Could you check a few things on this model? Use its own coordinates, in mm. Round coordinates to 2 decimals unless told otherwise and drop trailing zeros. Write each loop counter-clockwise with the first axis right and the second up, starting at its lowest first coordinate (ties: lowest second). Pieces come first, ordered by that corner, then holes. Notation, with made-up numbers: (31, 48.5) - (83, 48.5) arc R15 ccw to (83, 56.5) - close; hole circle Ø9 at (-39, 80.5). An arc over 180 degrees is marked (long way). Write each question's results on one line, items separated by ' | '. Start each with the question number.
(1) Imagine slicing it at B-B on z = 2.2. State how many separate pieces and enclosed holes the cut face has, then the cut area to 3 significant figures.
(2) Please list where these lines run through material, in increasing order: line 1 (X direction, y = -50.5, z = 1.2); line 2 (X direction, y = 9, z = 2.4); line 3 (Y direction, x = 144, z = 0.4). Write a range as [from, to].
(3) Imagine slicing it at A-A on y = 17. Write out the boundary of the cut face in (x, z), then the cut area to 3 significant figures.
(4) Thinking about a two-plate mould opening in X: for faces 1 (the cylindrical face through (42.734, -25.896, 1.972)), 2 (the flat face through (73, -15, 4)), which applies, +X half, -X half, draft (parallel to the pull), parting line (faces both ways), or undercut?
```python
from build123d import *

# Parameters (mm, degrees)
SKETCH1_W           = 270
SKETCH1_H           = 200
SKETCH1_R           = 1.5
SKETCH1_R_2         = 10
SKETCH1_R_3         = 2.5
BOSS_EXTRUDE1_DEPTH = 4


with BuildPart() as part:
    # Sketch1 → Boss-Extrude1 (new body)
    with BuildSketch(Plane.XY):
        with Locations((74.901502586, -16.133333333)):
            Rectangle(SKETCH1_W, SKETCH1_H)
        with Locations((-32.098497414, -92.133333333)):
            Circle(SKETCH1_R, mode=Mode.SUBTRACT)
        with Locations((-17.098497414, -92.133333333)):
            Circle(SKETCH1_R, mode=Mode.SUBTRACT)
        with Locations((-32.098497414, -107.133333333)):
            Circle(SKETCH1_R, mode=Mode.SUBTRACT)
        with Locations((-47.098497414, -92.133333333)):
            Circle(SKETCH1_R, mode=Mode.SUBTRACT)
        with Locations((-32.098497414, -77.133333333)):
            Circle(SKETCH1_R, mode=Mode.SUBTRACT)
        with Locations((74.901502586, -16.133333333)):
            Circle(SKETCH1_R, mode=Mode.SUBTRACT)
        with Locations((196.901502586, -92.133333333)):
            Circle(SKETCH1_R, mode=Mode.SUBTRACT)
        with Locations((181.901502586, -77.133333333)):
            Circle(SKETCH1_R, mode=Mode.SUBTRACT)
        with Locations((181.901502586, -92.133333333)):
            Circle(SKETCH1_R, mode=Mode.SUBTRACT)
        with Locations((181.901502586, -107.133333333)):
            Circle(SKETCH1_R, mode=Mode.SUBTRACT)
        with Locations((166.901502586, -92.133333333)):
            Circle(SKETCH1_R, mode=Mode.SUBTRACT)
        with Locations((196.901502586, 59.866666667)):
            Circle(SKETCH1_R, mode=Mode.SUBTRACT)
        with Locations((181.901502586, 74.866666667)):
            Circle(SKETCH1_R, mode=Mode.SUBTRACT)
        with Locations((181.901502586, 59.866666667)):
            Circle(SKETCH1_R, mode=Mode.SUBTRACT)
        with Locations((181.901502586, 44.866666667)):
            Circle(SKETCH1_R, mode=Mode.SUBTRACT)
        with Locations((166.901502586, 59.866666667)):
            Circle(SKETCH1_R, mode=Mode.SUBTRACT)
        with Locations((-17.098497414, 59.866666667)):
            Circle(SKETCH1_R, mode=Mode.SUBTRACT)
        with Locations((-32.098497414, 74.866666667)):
            Circle(SKETCH1_R, mode=Mode.SUBTRACT)
        with Locations((-32.098497414, 59.866666667)):
            Circle(SKETCH1_R, mode=Mode.SUBTRACT)
        with Locations((-32.098497414, 44.866666667)):
            Circle(SKETCH1_R, mode=Mode.SUBTRACT)
        with Locations((-47.098497414, 59.866666667)):
            Circle(SKETCH1_R, mode=Mode.SUBTRACT)
        with Locations((181.901502586, -16.133333333)):
            Circle(SKETCH1_R, mode=Mode.SUBTRACT)
        with Locations((74.901502586, 59.866666667)):
            Circle(SKETCH1_R, mode=Mode.SUBTRACT)
        with Locations((104.901502586, -16.133333333)):
            Circle(SKETCH1_R_2, mode=Mode.SUBTRACT)
        with Locations((44.901502586, -16.133333333)):
            Circle(SKETCH1_R_2, mode=Mode.SUBTRACT)
        with Locations((-32.098497414, -16.133333333)):
            Circle(SKETCH1_R, mode=Mode.SUBTRACT)
        with Locations((74.901502586, -92.133333333)):
            Circle(SKETCH1_R, mode=Mode.SUBTRACT)
        with Locations((4.901502586, 38.866666667)):
            Circle(SKETCH1_R_3, mode=Mode.SUBTRACT)
        with Locations((54.901502586, 38.866666667)):
            Circle(SKETCH1_R_3, mode=Mode.SUBTRACT)
        with Locations((94.901502586, 38.866666667)):
            Circle(SKETCH1_R_3, mode=Mode.SUBTRACT)
        with Locations((144.901502586, 38.866666667)):
            Circle(SKETCH1_R_3, mode=Mode.SUBTRACT)
        with Locations((94.901502586, -71.133333333)):
            Circle(SKETCH1_R_3, mode=Mode.SUBTRACT)
        with Locations((144.901502586, -71.133333333)):
            Circle(SKETCH1_R_3, mode=Mode.SUBTRACT)
        with Locations((4.901502586, -71.133333333)):
            Circle(SKETCH1_R_3, mode=Mode.SUBTRACT)
        with Locations((54.901502586, -71.133333333)):
            Circle(SKETCH1_R_3, mode=Mode.SUBTRACT)
        with Locations((-45.098497414, 8.866666667)):
            Circle(SKETCH1_R, mode=Mode.SUBTRACT)
        with Locations((12.901502586, 8.866666667)):
            Circle(SKETCH1_R, mode=Mode.SUBTRACT)
        with Locations((12.901502586, -40.133333333)):
            Circle(SKETCH1_R, mode=Mode.SUBTRACT)
        with Locations((-45.098497414, -40.133333333)):
            Circle(SKETCH1_R, mode=Mode.SUBTRACT)
        with Locations((29.901502586, 35.366666667)):
            Circle(SKETCH1_R, mode=Mode.SUBTRACT)
        with Locations((87.901502586, 35.366666667)):
            Circle(SKETCH1_R, mode=Mode.SUBTRACT)
        with Locations((87.901502586, -67.633333333)):
            Circle(SKETCH1_R, mode=Mode.SUBTRACT)
        with Locations((29.901502586, -67.633333333)):
            Circle(SKETCH1_R, mode=Mode.SUBTRACT)
        with Locations((107.901502586, 33.866666667)):
            Circle(SKETCH1_R, mode=Mode.SUBTRACT)
        with Locations((187.901502586, 33.866666667)):
            Circle(SKETCH1_R, mode=Mode.SUBTRACT)
        with Locations((187.901502586, -66.133333333)):
            Circle(SKETCH1_R, mode=Mode.SUBTRACT)
        with Locations((107.901502586, -66.133333333)):
            Circle(SKETCH1_R, mode=Mode.SUBTRACT)
        with BuildLine():
            Line((183.401502586, -45.133333333), (183.401502586, -73.133333333))
            ThreePointArc((183.401502586, -73.133333333), (181.901502586, -74.633333333), (180.401502586, -73.133333333))
            Line((180.401502586, -73.133333333), (180.401502586, -45.133333333))
            ThreePointArc((180.401502586, -45.133333333), (181.901502586, -43.633333333), (183.401502586, -45.133333333))
        make_face(mode=Mode.SUBTRACT)
        with BuildLine():
            Line((-33.598497414, -45.133333333), (-33.598497414, -73.133333333))
            ThreePointArc((-33.598497414, -73.133333333), (-32.098497414, -74.633333333), (-30.598497414, -73.133333333))
            Line((-30.598497414, -73.133333333), (-30.598497414, -45.133333333))
            ThreePointArc((-30.598497414, -45.133333333), (-32.098497414, -43.633333333), (-33.598497414, -45.133333333))
        make_face(mode=Mode.SUBTRACT)
        with BuildLine():
            Line((-33.598497414, 40.866666667), (-33.598497414, 12.866666667))
            ThreePointArc((-33.598497414, 12.866666667), (-32.098497414, 11.366666667), (-30.598497414, 12.866666667))
            Line((-30.598497414, 12.866666667), (-30.598497414, 40.866666667))
            ThreePointArc((-30.598497414, 40.866666667), (-32.098497414, 42.366666667), (-33.598497414, 40.866666667))
        make_face(mode=Mode.SUBTRACT)
        with BuildLine():
            Line((180.401502586, 40.866666667), (180.401502586, 12.866666667))
            ThreePointArc((180.401502586, 12.866666667), (181.901502586, 11.366666667), (183.401502586, 12.866666667))
            Line((183.401502586, 12.866666667), (183.401502586, 40.866666667))
            ThreePointArc((183.401502586, 40.866666667), (181.901502586, 42.366666667), (180.401502586, 40.866666667))
        make_face(mode=Mode.SUBTRACT)
    extrude(amount=BOSS_EXTRUDE1_DEPTH)


solid = part.part
```
Response:
1) separate pieces: 1 | enclosed holes: 51 | area: 52,600 mm²
2) line 1: [-60.1, -33.6], [-30.6, 180.4], [183.4, 209.9] | line 2: [-60.1, -46.59], [-43.6, 11.41], [14.4, 209.9] | line 3: [-116.13, -73.47], [-68.8, 36.53], [41.2, 83.87]
3) outline: (-60.1, 0) - (-33.6, 0) - (-33.6, 4) - (-60.1, 4) - close; (-30.6, 0) - (180.4, 0) - (180.4, 4) - (-30.6, 4) - close; (183.4, 0) - (209.9, 0) - (209.9, 4) - (183.4, 4) - close | area: 1,060 mm²
4) face 1: undercut | face 2: draft
